Geometry check sheet. Reference: drawing and pictorial views, mm from the part's lowest x, y, z. A direction names the side the tool comes from. Coordinates: 2 decimals unless noted, no trailing zeros. Write each loop counter-clockwise with the first axis right and the second up, starting at its lowest first coordinate (ties: lowest second). Pieces come first, ordered by that corner, then holes. Notation, with made-up numbers: (16, -24.5) -> (62, -24.5) arc R9 ccw to (62, -16.5) -> close; hole circle Ø3 at (-26.5, 42). An arc over 180 degrees is marked (long way). Put each result on its own line as item: value.
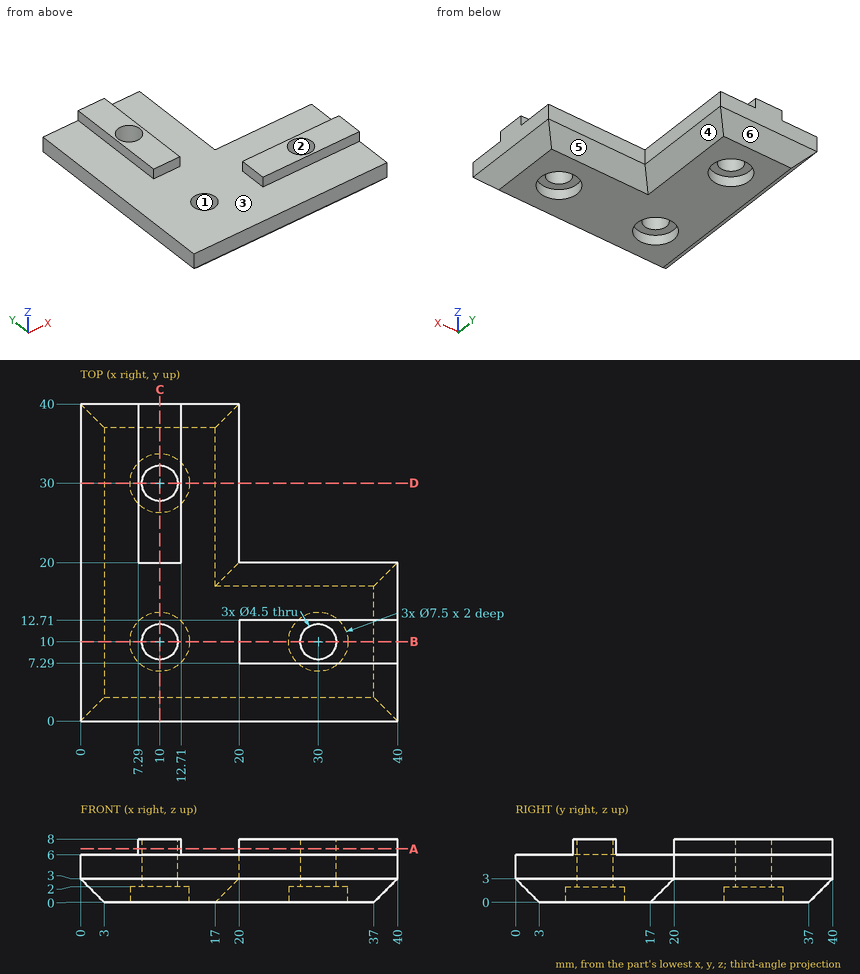
Q1. Cross-section at A-A (z = 6.75). Record the cut outline in (x, y), plus the area to 3 significant figures.
Recorded:
outline: (7.29, 20) -> (12.71, 20) -> (12.71, 40) -> (7.29, 40) -> close; (20, 7.29) -> (40, 7.29) -> (40, 12.71) -> (20, 12.71) -> close; hole circle Ø4.5 at (10, 30); hole circle Ø4.5 at (30, 10)
area: 185 mm2
Q2. Material ranges on line 1 along Y through (x, z) = (10, 4.9); line 2 along X through (y, z) = (30, 4.05), recorded low to high.
Recorded:
line 1: y = 0 to 7.75, 12.25 to 27.75, 32.25 to 40
line 2: x = 0 to 7.75, 12.25 to 20
Q3. Mould release check, pull along X, two halves, no side actions. Record for the marked faces 1, 2, 3 and 4: released by +X, released by -X, zero draft, split by the parting line, or undercut.
Recorded:
face 1: undercut
face 2: undercut
face 3: zero draft
face 4: released by +X
Q4. Cross-section at D-D (y = 30). Record the cut outline in (x, z).
Recorded:
outline: (0, 3) -> (3, 0) -> (6.25, 0) -> (6.25, 2) -> (7.75, 2) -> (7.75, 8) -> (7.29, 8) -> (7.29, 6) -> (0, 6) -> close; (12.25, 2) -> (13.75, 2) -> (13.75, 0) -> (17, 0) -> (20, 3) -> (20, 6) -> (12.71, 6) -> (12.71, 8) -> (12.25, 8) -> close
Q5. Depth check by flat-ended pin: P1, Ø0.6, axis at x = 10.5, z = 6.5, coming from the -Y side; P2, Ø1.5, axis at x = 34, z = 1.5, coming from the -Y side; P3, Ø1, axis at x = 28.5, z = 4.5, coming from the +Y side. Enter the tip coordinate at first touch or a pass-through.
Recorded:
P1: stops at y = 20
P2: stops at y = 0.75
P3: stops at y = 20
Q6. Cross-section at B-B (y = 10). Record the cut outline in (x, z).
Recorded:
outline: (0, 3) -> (3, 0) -> (6.25, 0) -> (6.25, 2) -> (7.75, 2) -> (7.75, 6) -> (0, 6) -> close; (12.25, 2) -> (13.75, 2) -> (13.75, 0) -> (26.25, 0) -> (26.25, 2) -> (27.75, 2) -> (27.75, 8) -> (20, 8) -> (20, 6) -> (12.25, 6) -> close; (32.25, 2) -> (33.75, 2) -> (33.75, 0) -> (37, 0) -> (40, 3) -> (40, 8) -> (32.25, 8) -> close
Q7. Tool access check on the marked faces 5 and 6. Record the directions out of +Z, -Z, +X, -X, +Y, -Y that give a thin tool (end or side, any length) a straight path to the whole face; none if there is none.
Recorded:
face 5: -Z, +X, +Y
face 6: -Z, +X, -X, +Y
